Autodesk Fusion 360 part; units mm, degrees
sketch "Sketch1" plane through (0, 0, 0) normal (0, 0, 1) x (1, 0, 0)
  line L0 (33, -21) -> (-33, -21)
  line L1 (-33, -21) -> (-33, 21)
  line L2 (-33, 21) -> (33, 21)
  line L3 (33, 21) -> (33, -21)
  line L4 (33, -21) -> (-33, 21) construction
  line L5 (-33, -21) -> (33, 21) construction
  dimension "d1" = 66
  dimension "d2" = 42
extrude "Extrude1" add sketch "Sketch1" along normal blind 12
chamfer "Chamfer1" distance 12 angle 45 2 edges at (33, 21, 6) (33, -21, 6)
sketch "Sketch2" plane through (0, 0, 12) normal (0, 0, 1) x (-1, 0, 0)
  line L0 (-21, 21) -> (-33, 9)
  line L1 (-33, 9) -> (-33, -9)
  line L2 (-33, -9) -> (-21, -21)
  line L3 (-21, -21) -> (33, -21)
  line L4 (33, -21) -> (33, 21)
  line L5 (33, 21) -> (-21, 21)
  line L6 (33, -21) -> (21, -21)
  line L7 (21, -21) -> (21, 21)
  line L8 (21, 21) -> (33, 21)
  line L9 (33, 21) -> (33, -21)
  dimension "d6" = 12
extrude "Extrude2" add sketch "Sketch2" along normal blind 48 contours L3 L4 L5 L6 L7 L8 L9
fillet "Fillet1" radius 21 2 edges at (-27, -21, 60) (-27, 21, 60)
sketch "Sketch3" plane through (0, 0, 12) normal (0, 0, 1) x (-1, 0, 0)
  line L0 (21, -21) -> (21, 21)
  line L1 (21, 21) -> (-21, 21)
  line L2 (-21, 21) -> (-33, 9)
  line L3 (-33, 9) -> (-33, -9)
  line L4 (-33, -9) -> (-21, -21)
  line L5 (-21, -21) -> (21, -21)
sketch "Sketch4" plane through (0, 0, 0) normal (0, 1, 0) x (1, 0, 0)
  line L0 (-21.0093, -54.0965) -> (-21.0093, -12.0965)
  line L1 (-21.0093, -12.0965) -> (32.9907, -12.0965)
  line L2 (32.9907, -12.0965) -> (-21.0093, -54.0965)
  dimension "d10" = 42
  dimension "d11" = 54
extrude "Extrude3" add sketch "Sketch4" along normal mid plane 12
equation "d7 = 60 mm - 12 mm"
equation "d11 = 66 mm - 12 mm"
Could you check a few things on this model? Use its own coordinates, in mm. A direction names the side the tool comes from. Give positions to 0.01 mm unless a question says otherwise; leave off trailing zeros. Write each loop counter-clockwise with the first axis right and the second up, starting at its lowest first coordinate (ties: lowest second). Pieces come first, ordered by that corner, then holes. Notation, with made-up numbers: (1.5, 73) - (52.5, 73) arc R15 ccw to (52.5, 81) - close; hole circle Ø2 at (-29.75, 32.5). An arc over 180 degrees is marked (long way). Use CSV: the item, a comma, the result in double quotes. Start each with the question number.
Item 1: For faces 1 (the face through (0, 6, 28)), 2 (the face through (-12, -21, 11)), 3 (the face through (0, -6, 28)), which set-ups out of +Z, -Z, +X, -X, +Y, -Y let a thin tool reach every point of the face, with its end or its side?
Item 2: I want a section at B-B, the plane z = 22.5. Please give me the cut outline in (x, y).
Item 3: I want a section at C-C, the plane y = -3. Please give me the cut outline in (x, z).
Item 4: If I drill on line 1 along Y through (x, z) = (15.5, 16); line 2 along Z through (x, y) = (-18.5, -10); line 3 along X through (y, z) = (16.5, 49), over which ranges is the centre line in solid material (lowest first)?
Item 5: I'm going to push flat-ended pins straight in: pin 1 (3 mm diameter, centred on y = 6, z = 44, fed in from +X); pin 2 (2 mm diameter, centred on y = 8.5, z = 31.5, fed in from +X); pin 3 (12.5 mm diameter, centred on x = 7, z = 35, fed in from -Y). Where does each tip first touch, or does it pass through?
Item 6: I want a section at A-A, the plane x = -15. Please give me the cut outline in (y, z), then the cut area to 3 significant figures.
Item 7: I want a section at D-D, the plane x = 29. Please give me the cut outline in (y, z).
Findings:
1,face 1,"+Z, +X, +Y"
1,face 2,"+Z, -Z, +X, -X, -Y"
1,face 3,"+Z, +X, -Y"
2,outline,"(-33, -21) - (-21, -21) - (-21, -6) - (19.61, -6) - (19.61, 6) - (-21, 6) - (-21, 21) - (-33, 21) - close"
3,outline,"(-33, 0) - (33, 0) - (33, 12) - (-21, 12) - (-21, 12.1) - (32.99, 12.1) - (-21, 54.09) - (-21, 59.79) - (-33, 59.79) - close"
4,line 1,"y = -6 to 6"
4,line 2,"z = 0 to 12"
4,line 3,"x = -33 to -21"
5,pin 1,"stops at x = -6.1"
5,pin 2,"stops at x = -21"
5,pin 3,"stops at y = -6"
6,outline,"(-21, 0) - (21, 0) - (21, 12) - (-21, 12) - close; (-6, 12.1) - (6, 12.1) - (6, 49.42) - (-6, 49.42) - close"
6,area,"952 mm2"
7,outline,"(-13, 0) - (13, 0) - (13, 12) - (-13, 12) - close; (-6, 12.1) - (6, 12.1) - (6, 15.2) - (-6, 15.2) - close"
